Build history of the part. All positions in model axes, mm. Face numbers are marked on the shaded views. A direction names the side the tool comes from. Round coordinates to 2 decimals unless told otherwise and drop trailing zeros. Order: outer loops, then holes, each group sorted by start corner. A loop starts at its lowest first (then second) coordinate and runs counter-clockwise, first axis right, second up. Notation, with made-up numbers: (56.5, -20.75) -> (62.5, -20.75) arc R22 ccw to (62.5, -0.75) -> close; hole circle Ø11 at (77.25, 83). An arc over 180 degrees is marked (long way). Write item = value, one per line.
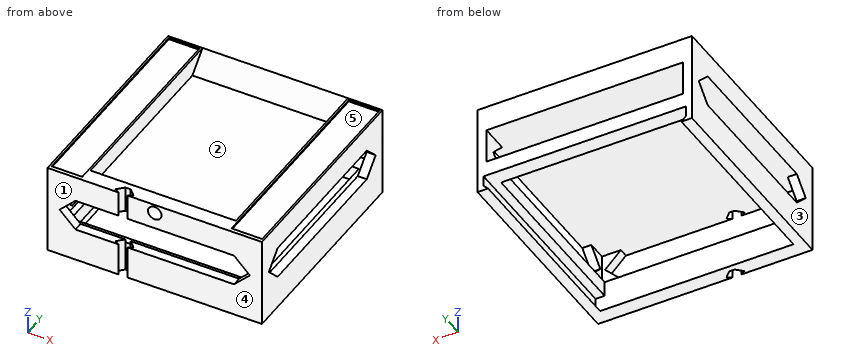
from build123d import *

# Parameters (mm, degrees)
SKETCH1_W            = 142
SKETCH1_H            = 142
SKETCH1_W_2          = 122
SKETCH1_H_2          = 122
BOSS_EXTRUDE1_DEPTH  = 10
SKETCH2_W            = 142
SKETCH2_H            = 10
BOSS_EXTRUDE2_DEPTH  = 10
BOSS_EXTRUDE3_DEPTH  = 132
BOSS_EXTRUDE4_DEPTH  = 2
SKETCH6_W            = 6
SKETCH6_H            = 8
BOSS_EXTRUDE5_DEPTH  = 21
BOSS_EXTRUDE6_DEPTH  = 142
BOSS_EXTRUDE7_DEPTH  = 6
BOSS_EXTRUDE8_DEPTH  = 6
SKETCH10_W           = 142
SKETCH10_H           = 142
BOSS_EXTRUDE9_DEPTH  = 12
BOSS_EXTRUDE14_DEPTH = 6
SKETCH13_R           = 4.5
CUT_EXTRUDE2_DEPTH   = 159.003164525
SKETCH14_W           = 20.32
SKETCH14_H           = 138.19
CUT_EXTRUDE3_DEPTH   = 1
CHAMFER4_SIZE        = 12
CUT_EXTRUDE4_DEPTH   = 117.970081645


with BuildPart() as part:
    # Sketch1 → Boss-Extrude1 (new body)
    with BuildSketch(Plane(origin=(0, 0, 0), x_dir=(0, 1, 0), z_dir=(0, 0, 1))):
        Rectangle(SKETCH1_W, SKETCH1_H)
        Rectangle(SKETCH1_W_2, SKETCH1_H_2, mode=Mode.SUBTRACT)
    extrude(amount=BOSS_EXTRUDE1_DEPTH)

    # Sketch2 → Boss-Extrude2 (add)
    with BuildSketch(Plane(origin=(0, 0, 0), x_dir=(1, 0, 0), z_dir=(0, 0, -1))):
        with Locations((0, 66)):
            Rectangle(SKETCH2_W, SKETCH2_H)
    extrude(amount=BOSS_EXTRUDE2_DEPTH)

    # Sketch3 → Boss-Extrude3 (add)
    with BuildSketch(Plane(origin=(0, -61, 0), x_dir=(-1, 0, 0), z_dir=(0, 1, 0))):
        Polygon((-67, -7), (-64, -10), (-71, -10), (-71, 0), (-67, 0), align=None)
        Polygon((64, -10), (71, -10), (71, 0), (67, 0), (67, -7), align=None)
    extrude(amount=BOSS_EXTRUDE3_DEPTH)

    # Sketch5 → Boss-Extrude4 (add)
    with BuildSketch(Plane.XY.offset(10)):
        Polygon((-65, -65), (65, -65), (65, 65), (65, 71), (71, 71), (71, 65), (71, -71), (-71, -71), (-71, 71), (-65, 71), (-65, 65), align=None)
    extrude(amount=BOSS_EXTRUDE4_DEPTH)

    # Sketch6 → Boss-Extrude5 (add)
    with BuildSketch(Plane.XY.offset(12)):
        with Locations((-68, 67)):
            Rectangle(SKETCH6_W, SKETCH6_H)
        Polygon((-65, -65), (-65, -63), (-71, -63), (-71, -71), (-63, -71), (-63, -65), align=None)
        Polygon((63, -71), (63, -65), (65, -65), (65, -63), (71, -63), (71, -71), align=None)
        with Locations((68, 67)):
            Rectangle(SKETCH6_W, SKETCH6_H)
    extrude(amount=BOSS_EXTRUDE5_DEPTH)

    # Sketch7 → Boss-Extrude6 (add)
    with BuildSketch(Plane.XZ.offset(71)):
        Polygon((-63, 33), (63, 33), (71, 33), (71, 38), (-71, 38), (-71, 33), align=None)
    extrude(amount=-BOSS_EXTRUDE6_DEPTH)

    # Sketch8 → Boss-Extrude7 (add)
    with BuildSketch(Plane.YZ.offset(71)):
        Polygon((63, 12), (63, 22.5), (52.5, 12), align=None)
        Polygon((52.5, 33), (63, 22.5), (63, 33), align=None)
    boss_extrude7 = extrude(amount=-BOSS_EXTRUDE7_DEPTH)

    # Sketch9 → Boss-Extrude8 (add)
    with BuildSketch(Plane(origin=(-71, 0, 0), x_dir=(0, -1, 0), z_dir=(-1, 0, 0))):
        Polygon((-52.5, 12), (-63, 22.5), (-63, 12), align=None)
        Polygon((-52.5, 33), (-63, 33), (-63, 22.5), align=None)
    boss_extrude8 = extrude(amount=-BOSS_EXTRUDE8_DEPTH)

    # Mirror4: Boss-Extrude7, Boss-Extrude8 across plane
    add(boss_extrude7.mirror(Plane.ZX))
    add(boss_extrude8.mirror(Plane.ZX))

    # Sketch10 → Boss-Extrude9 (add)
    with BuildSketch(Plane.XY.offset(38)):
        Rectangle(SKETCH10_W, SKETCH10_H)
        Polygon((-48.14, 59), (-48.14, -48.14), (-48.14, -61), (48.14, -61), (48.14, -48.14), (48.14, 59), align=None, mode=Mode.SUBTRACT)
    extrude(amount=BOSS_EXTRUDE9_DEPTH)

    # Sketch11 → Boss-Extrude14 (add)
    with BuildSketch(Plane.XZ.offset(71)):
        Polygon((-52.5, 12), (-63, 22.5), (-63, 12), align=None)
        Polygon((-63, 33), (-63, 22.5), (-52.5, 33), align=None)
    boss_extrude14 = extrude(amount=-BOSS_EXTRUDE14_DEPTH)

    # Mirror5: Boss-Extrude14 across plane
    add(boss_extrude14.mirror(Plane(origin=(0, 0, 0), x_dir=(0, 0, 1), z_dir=(1, 0, 0))))

    # Sketch13 → Cut-Extrude2 (cut, through all)
    with BuildSketch(Plane(origin=(0, -61, 0), x_dir=(-1, 0, 0), z_dir=(0, 1, 0))):
        with Locations(Location((0, 44, 0), (0, 0, 90))):
            Circle(SKETCH13_R)
    extrude(amount=-CUT_EXTRUDE2_DEPTH, mode=Mode.SUBTRACT)

    # Sketch14 → Cut-Extrude3 (cut)
    with BuildSketch(Plane.XY.offset(50)):
        with Locations((-59.57, 0.635)):
            Rectangle(SKETCH14_W, SKETCH14_H)
        with Locations((59.57, 0.635)):
            Rectangle(SKETCH14_W, SKETCH14_H)
    extrude(amount=-CUT_EXTRUDE3_DEPTH, mode=Mode.SUBTRACT)

    # Chamfer4
    chamfer4_edges = [part.edges().sort_by_distance(p)[0] for p in [
        (0, 59, 50),
    ]]
    chamfer(chamfer4_edges, length=CHAMFER4_SIZE - 0.0001)  # a hair under: the kernel refuses the full size

    # Sketch15 → Cut-Extrude4 (cut, through all)
    with BuildSketch(Plane.XY.offset(50)):
        Polygon((-24, -71), (-18, -71), (-15, -69.254896882), (-19.254896882, -65), (-22.745103118, -65), (-27, -69.254896882), align=None)
    extrude(amount=-CUT_EXTRUDE4_DEPTH, mode=Mode.SUBTRACT)


solid = part.part
Q1. Which spindle directions (+Z, -Z, +X, -X, +Y, -Y) get a long thin tool onto all of the face, cutting with end or side? Do the marked faces 1 and 2. Say none if no direction does.
Check values:
face_1 = +Z, -Z, +X, -X, -Y
face_2 = +Z
Q2. Mould opens along Y. For the marked faces 3, 4 and 5 say: released by +Y, released by -Y, zero draft, split by the parting line, or undercut.
Check values:
face_3 = zero draft
face_4 = released by -Y
face_5 = undercut
Q3. Cut at B-B, the plane z = 6. List the corners of the cut face in (x, y).
Check values:
outline = (-71, -71) -> (-24, -71) -> (-27, -69.25) -> (-22.75, -65) -> (-19.25, -65) -> (-15, -69.25) -> (-18, -71) -> (71, -71) -> (71, 71) -> (-71, 71) -> close; hole (-61, -61) -> (61, -61) -> (61, 61) -> (-61, 61) -> close
Q4. Cut at A-A, the plane y = 49.5. Give the number of separate pieces and of enclosed holes in the cut face, and give its area (3 significant figures).
Check values:
separate_pieces = 3
enclosed_holes = 0
area = 1,530 mm²
Q5. Flat gauge pins, fed straight in: pin 1 (1.5 mm diameter, centred on x = 55.5, y = 5, fed in from -Z); pin 2 (1.5 mm diameter, centred on x = -13.5, y = -19, fed in from +Z); pin 3 (4 mm diameter, centred on x = -21, z = 2, fed in from -Y); pin 4 (22 mm diameter, centred on x = 14.5, z = -3.5, fed in from +Y). Where does each tip first touch, or does it go through?
Check values:
pin_1 = 33
pin_2 = 38
pin_3 = -65.25
pin_4 = 71
Q6. Probe probe 1 along X at (y, z) = (47.5, 9); probe 2 along X at (y, z) = (-63.25, 44). List the from-to ranges inside material, lowest first.
Check values:
probe_1 = -71 to -61, 61 to 71
probe_2 = -71 to -4.5, 4.5 to 71
